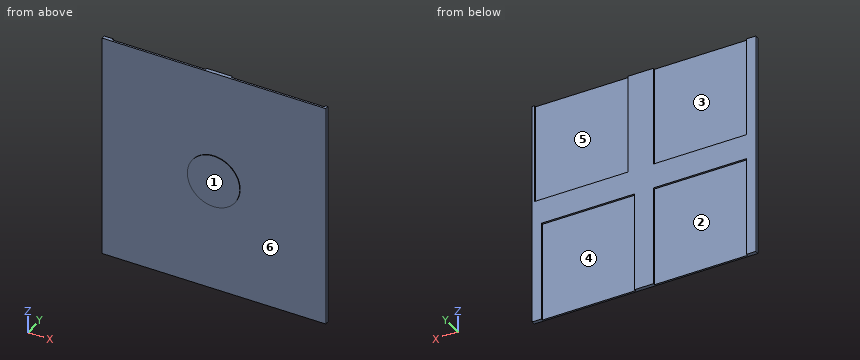
from build123d import *

# Parameters (mm, degrees)
SKETCH_1_W          = 360
SKETCH_1_H          = 360
EXTRUDE_1_DEPTH     = 6
SKETCH_2_W          = 140
SKETCH_2_H          = 140
CUT_EXTRUDE_1_DEPTH = 3
SKETCH_7_W          = 140
SKETCH_7_H          = 169.149624319
CUT_EXTRUDE_2_DEPTH = 110
SKETCH_4_R          = 42.212172728
EXTRUDE_2_DEPTH     = 1
SKETCH_10_W         = 6
SKETCH_10_H         = 160
CUT_EXTRUDE_3_DEPTH = 3
SKETCH_11_W         = 6
SKETCH_11_H         = 160
EXTRUDE_3_DEPTH     = 3
SKETCH_12_W         = 14
SKETCH_12_H         = 160
CUT_EXTRUDE_4_DEPTH = 3
SKETCH_13_W         = 14
SKETCH_13_H         = 160
EXTRUDE_4_DEPTH     = 3
SKETCH_14_W         = 4
SKETCH_14_H         = 160
EXTRUDE_5_DEPTH     = 3
SKETCH_15_W         = 4
SKETCH_15_H         = 160
CUT_EXTRUDE_5_DEPTH = 3
CUT_EXTRUDE_6_DEPTH = 3
SKETCH_17_W         = 150
SKETCH_17_H         = 165.602098182
CUT_EXTRUDE_7_DEPTH = 3


with BuildPart() as part:
    # 草图1 → 凸台-拉伸1 (new body)
    with BuildSketch(Plane(origin=(0, 0, 0), x_dir=(1, 0, 0), z_dir=(0, 1, 0))):
        Rectangle(SKETCH_1_W, SKETCH_1_H)
    extrude(amount=EXTRUDE_1_DEPTH)

    # 草图2 → 切除-拉伸1 (cut)
    with BuildSketch(Plane(origin=(0, 6, 0), x_dir=(1, 0, 0), z_dir=(0, 1, 0))):
        with Locations((-90, -90)):
            Rectangle(SKETCH_2_W, SKETCH_2_H)
        with Locations((90, -90)):
            Rectangle(SKETCH_2_W, SKETCH_2_H)
        with Locations((90, 90)):
            Rectangle(SKETCH_2_W, SKETCH_2_H)
        with Locations((-90, 90)):
            Rectangle(SKETCH_2_W, SKETCH_2_H)
    extrude(amount=-CUT_EXTRUDE_1_DEPTH, mode=Mode.SUBTRACT)

    # 草图7 → 切除-拉伸2 (cut)
    with BuildSketch(Plane(origin=(0, 3, 0), x_dir=(1, 0, 0), z_dir=(0, 1, 0))):
        with Locations((90, -104.57481216)):
            Rectangle(SKETCH_7_W, SKETCH_7_H)
        with Locations((-90, -104.57481216)):
            Rectangle(SKETCH_7_W, SKETCH_7_H)
        with Locations((90, 104.57481216)):
            Rectangle(SKETCH_7_W, SKETCH_7_H)
        with Locations((-90, 104.57481216)):
            Rectangle(SKETCH_7_W, SKETCH_7_H)
    extrude(amount=CUT_EXTRUDE_2_DEPTH, mode=Mode.SUBTRACT)

    # 草图4 → 凸台-拉伸2 (add)
    with BuildSketch(Plane.XZ):
        with Locations(Location((0, 0, 0), (0, 0, 270))):
            Circle(SKETCH_4_R)
    extrude(amount=EXTRUDE_2_DEPTH)

    # 草图10 → 切除-拉伸3 (cut)
    with BuildSketch(Plane(origin=(0, 6, 0), x_dir=(1, 0, 0), z_dir=(0, 1, 0))):
        with Locations((163, -100)):
            Rectangle(SKETCH_10_W, SKETCH_10_H)
    extrude(amount=-CUT_EXTRUDE_3_DEPTH, mode=Mode.SUBTRACT)

    # 草图11 → 凸台-拉伸3 (add)
    with BuildSketch(Plane(origin=(0, 6, 0), x_dir=(1, 0, 0), z_dir=(0, 1, 0))):
        with Locations((23, -100)):
            Rectangle(SKETCH_11_W, SKETCH_11_H)
    extrude(amount=-EXTRUDE_3_DEPTH)

    # 草图12 → 切除-拉伸4 (cut)
    with BuildSketch(Plane(origin=(0, 6, 0), x_dir=(1, 0, 0), z_dir=(0, 1, 0))):
        with Locations((173, -100)):
            Rectangle(SKETCH_12_W, SKETCH_12_H)
    extrude(amount=-CUT_EXTRUDE_4_DEPTH, mode=Mode.SUBTRACT)

    # 草图13 → 凸台-拉伸4 (add)
    with BuildSketch(Plane(origin=(0, 3, 0), x_dir=(1, 0, 0), z_dir=(0, 1, 0))):
        with Locations((33, -100)):
            Rectangle(SKETCH_13_W, SKETCH_13_H)
    extrude(amount=EXTRUDE_4_DEPTH)

    # 草图14 → 凸台-拉伸5 (add)
    with BuildSketch(Plane(origin=(0, 3, 0), x_dir=(1, 0, 0), z_dir=(0, 1, 0))):
        with Locations((178, -100)):
            Rectangle(SKETCH_14_W, SKETCH_14_H)
    extrude(amount=EXTRUDE_5_DEPTH)

    # 草图15 → 切除-拉伸5 (cut)
    with BuildSketch(Plane(origin=(0, 6, 0), x_dir=(1, 0, 0), z_dir=(0, 1, 0))):
        with Locations((38, -100)):
            Rectangle(SKETCH_15_W, SKETCH_15_H)
    extrude(amount=-CUT_EXTRUDE_5_DEPTH, mode=Mode.SUBTRACT)

    # 草图16 → 切除-拉伸6 (cut)
    with BuildSketch(Plane(origin=(0, 6, 0), x_dir=(1, 0, 0), z_dir=(0, 1, 0))):
        Polygon((-15, -170), (-15, -20), (-165, -20), (-165, -170), (-165, -206.201346441), (-15, -206.201346441), align=None)
        Polygon((-165, 170), (-165, 20), (-15, 20), (-15, 170), (-15, 194.423731299), (-165, 194.423731299), align=None)
        Polygon((15, 170), (15, 194.423731299), (165, 194.423731299), (165, 170), (165, 20), (15, 20), align=None)
    extrude(amount=-CUT_EXTRUDE_6_DEPTH, mode=Mode.SUBTRACT)

    # 草图17 → 切除-拉伸7 (cut)
    with BuildSketch(Plane(origin=(0, 6, 0), x_dir=(1, 0, 0), z_dir=(0, 1, 0))):
        with Locations((101, -102.801049091)):
            Rectangle(SKETCH_17_W, SKETCH_17_H)
    extrude(amount=-CUT_EXTRUDE_7_DEPTH, mode=Mode.SUBTRACT)


solid = part.part
Work out the finished part from the listing and answer in its coordinate system (mm). Face numbers are marked on the shaded views. A direction names the side the tool comes from. Give positions to 0.01 mm unless a question says otherwise; leave off trailing zeros. Loops run counter-clockwise (first coordinate to the right, second up) from the corner with the lowest first, then second, coordinate; pieces in that order, holes last. Notation, with made-up numbers: (36.25, -39) -> (81.25, -39) arc R18 cw to (81.25, -10) -> close; hole circle Ø5 at (-9.5, 80). An arc over 180 degrees is marked (long way). Use a Markdown table: item, result. Add a question column.
1. Find the intervals of material crossed by probe 1 along X at (y, z) = (5, 95.5); probe 2 along X at (y, z) = (3.75, -113.5); probe 3 along Y at (x, z) = (138.5, 151.5), in increasing order.
2. Section C-C on x = 77.5 is taken. Determine the outline of the cut face in (y, z).
3. Flat-ended cylindrical pins translate along their axes: pin 1 Ø10 at (x, z) = (-38, 98) entering from +Y; pin 2 Ø1.5 at (x, y) = (-90.5, 4) entering from +Z; pin 3 Ø1.5 at (x, y) = (-65, 4.5) entering from -Z. Find the tip coordinate at first contact, or state that the pin passes through.
4. Section D-D on z = -127 is taken. Determine the outline of the cut face in (x, y), and give its area (3 significant figures).
5. Section B-B on y = 4.75 is taken. Determine the outline of the cut face in (x, z), and give its area (3 significant figures).
6. For the marked faces 1, 2 and 3, determine the directions among +Z, -Z, +X, -X, +Y, -Y from which every point of the face is accessible in a straight line to the end or side of a thin tool.
7. Determine the mould class of the marked faces 4, 5 and 6 for opening direction X: released by +X, released by -X, zero draft, split by the parting line, or undercut.
8. Section A-A on z = 0 is taken. Determine the outline of the cut face in (x, y), and give its area (3 significant figures).
Results below:
| question | item | result |
|---|---|---|
| 1 | probe 1 | x = -180 to -165, -15 to 26, 176 to 180 |
| 1 | probe 2 | x = -180 to -165, -15 to 15, 165 to 180 |
| 1 | probe 3 | y = 0 to 3 |
| 2 | outline | (0, -180) -> (3, -180) -> (3, -20) -> (6, -20) -> (6, 20) -> (3, 20) -> (3, 180) -> (0, 180) -> close |
| 3 | pin 1 | stops at y = 3 |
| 3 | pin 2 | stops at z = 20 |
| 3 | pin 3 | stops at z = -20 |
| 4 | outline | (-180, 0) -> (180, 0) -> (180, 6) -> (165, 6) -> (165, 3) -> (15, 3) -> (15, 6) -> (-15, 6) -> (-15, 3) -> (-165, 3) -> (-165, 6) -> (-180, 6) -> close |
| 4 | area | 1,260 mm^2 |
| 5 | outline | (-180, -180) -> (-165, -180) -> (-165, -20) -> (-15, -20) -> (-15, -180) -> (15, -180) -> (15, -20) -> (165, -20) -> (165, -180) -> (180, -180) -> (180, 180) -> (176, 180) -> (176, 20) -> (26, 20) -> (26, 180) -> (-15, 180) -> (-15, 20) -> (-165, 20) -> (-165, 180) -> (-180, 180) -> close |
| 5 | area | 33,600 mm^2 |
| 6 | face 1 | +Z, -Z, +X, -X, -Y |
| 6 | face 2 | -Z, +Y |
| 6 | face 3 | +Z, +Y |
| 7 | face 4 | undercut |
| 7 | face 5 | undercut |
| 7 | face 6 | zero draft |
| 8 | outline | (-180, 0) -> (-42.21, 0) -> (-42.21, -1) -> (42.21, -1) -> (42.21, 0) -> (180, 0) -> (180, 6) -> (-180, 6) -> close |
| 8 | area | 2,240 mm^2 |
